Geometry check sheet. Reference: drawing and pictorial views, mm from the part's lowest x, y, z. A direction names the side the tool comes from. Round coordinates to 2 decimals unless told otherwise and drop trailing zeros. Loops run counter-clockwise (first coordinate to the right, second up) from the corner with the lowest first, then second, coordinate; pieces in that order, holes last. Notation, with made-up numbers: (57, 32.25) - (66, 32.25) arc R35 ccw to (66, 65.25) - close; hole circle Ø1 at (30, 33.25). An arc over 180 degrees is marked (long way). Answer as CSV lines item,"result". Start each with the question number.
1) Thickness scan on line 1 along Z through (x, y) = (43, 7.75); line 2 along X through (y, z) = (7.5, 7); line 3 along Y through (x, z) = (5.5, 5.25). Record the ranges inside material, lowest first.
2) Cross-section at C-C on y = 5.25. Record the boundary of the cut face in (x, z), and give its area (3 significant figures).
3) Depth check by flat-ended pin: P1, Ø5.5, axis at y = 15.5, z = 10, coming from the +X side; P2, Ø2.5, axis at x = 25.5, y = 5, coming from the +Z side; P3, Ø8, axis at x = 49, y = 16, coming from the +Z side. Enter the tip coordinate at first touch or a pass-through.
4) Cross-section at D-D on z = 15. Record the boundary of the cut face in (x, y).
5) Cross-section at A-A on x = 44.5. Record the boundary of the cut face in (y, z).
6) Cross-section at B-B on z = 4.25. Record the boundary of the cut face in (x, y), and give its area (3 significant figures).
7) Access from +Z, -Z, +X, -X, +Y, -Y to the whole of each face (thin tool, end or side, straight path). Record for the marked faces 1, 2 and 3.
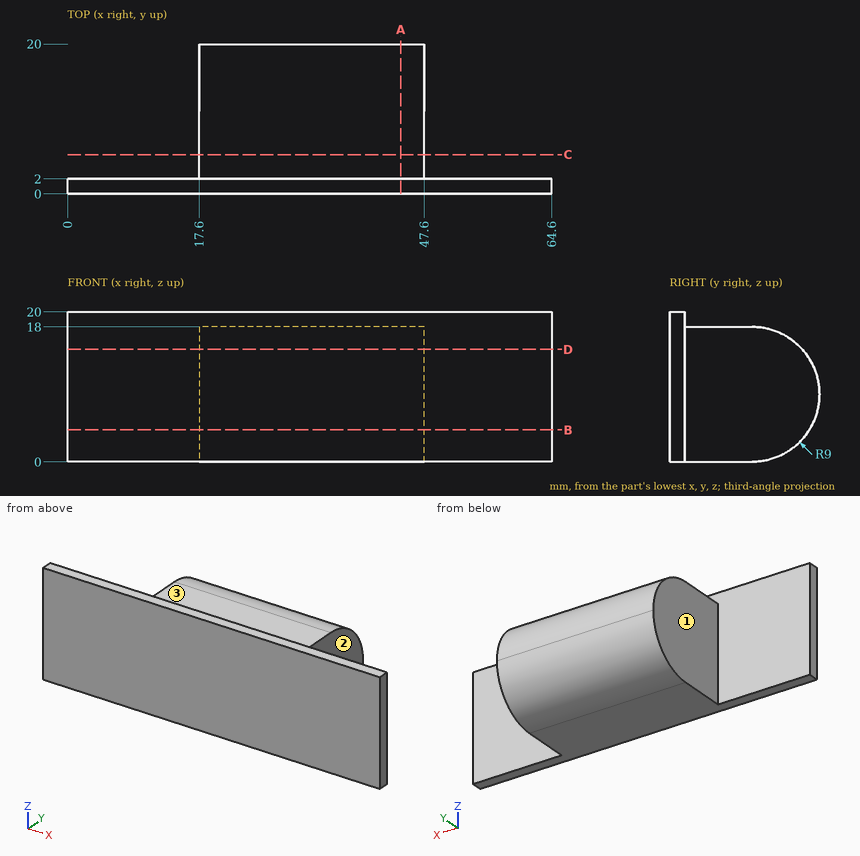
Answer block:
1,line 1,"z = 0 to 18"
1,line 2,"x = 17.6 to 47.6"
1,line 3,"y = 0 to 2"
2,outline,"(17.6, 0) - (47.6, 0) - (47.6, 18) - (17.6, 18) - close"
2,area,"540 mm^2"
3,P1,"stops at x = 47.6"
3,P2,"stops at z = 18"
3,P3,"stops at z = 17.91"
4,outline,"(0, 0) - (64.6, 0) - (64.6, 2) - (47.6, 2) - (47.6, 17.71) - (17.6, 17.71) - (17.6, 2) - (0, 2) - close"
5,outline,"(0, 0) - (11, 0) arc R9 ccw to (11, 18) - (2, 18) - (2, 20) - (0, 20) - close"
6,outline,"(0, 0) - (64.6, 0) - (64.6, 2) - (47.6, 2) - (47.6, 18.64) - (17.6, 18.64) - (17.6, 2) - (0, 2) - close"
6,area,"629 mm^2"
7,face 1,"+Z, -Z, -X, +Y"
7,face 2,"+Z, -Z, +X, +Y"
7,face 3,"+Z, +X, -X, +Y"
